The figure shows three views and two pictorial views of one solid part (mm, origin at its lowest corner). Answer the questions. A direction names the side the tool comes from. Coordinates: 2 decimals unless noted, no trailing zeros. Loops run counter-clockwise (first coordinate to the right, second up) from the corner with the lowest first, then second, coordinate; pieces in that order, holes last.
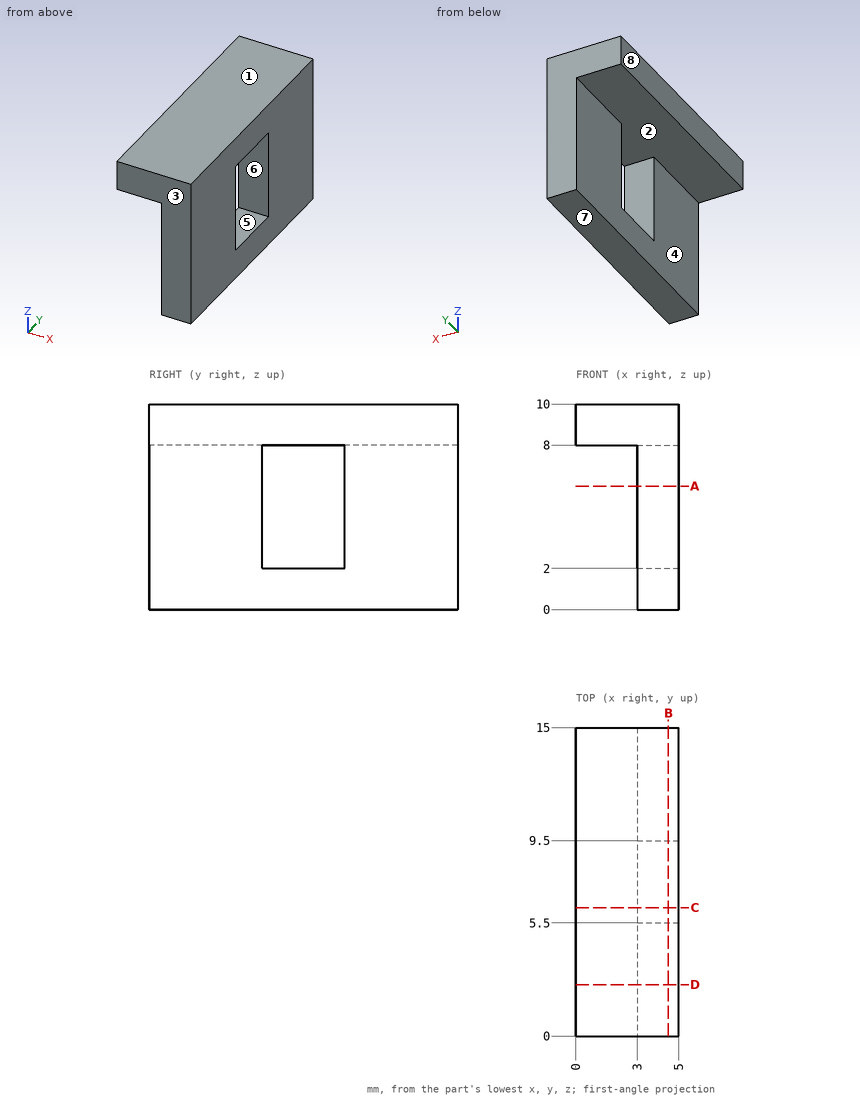
Q1. A cutting plane is placed at A-A (z = 6). Give the vertices of the cut face in (x, y).
Findings below:
outline: (3, 0) - (5, 0) - (5, 5.5) - (3, 5.5) - close; (3, 9.5) - (5, 9.5) - (5, 15) - (3, 15) - close
Q2. A cutting plane is placed at D-D (y = 2.5). Give the vertices of the cut face in (x, z), then the cut area to 3 significant figures.
Findings below:
outline: (0, 8) - (3, 8) - (3, 0) - (5, 0) - (5, 10) - (0, 10) - close
area: 26.0 mm2
Q3. Straight lines are drawn through the part: probe 1 along Y at (x, z) = (3.2, 4.5); probe 2 along X at (y, z) = (1.25, 4.5); probe 3 along Z at (x, y) = (2.95, 7.5). For each, find the intervals that lie inside material, in ascending order.
Findings below:
probe 1: y = 0 to 5.5, 9.5 to 15
probe 2: x = 3 to 5
probe 3: z = 8 to 10
Q4. Which of the six approach directions +Z, -Z, +X, -X, +Y, -Y give full straight-line access (tool end or side, diameter ignored) to the marked faces 1, 2, 3, 4 and 5?
Findings below:
face 1: +Z, +X, -X, +Y, -Y
face 2: -X
face 3: +Z, -Z, +X, -X, -Y
face 4: -Z, -X, +Y, -Y
face 5: +X, -X
Q5. A cutting plane is placed at B-B (x = 4.5). Give the vertices of the cut face in (y, z).
Findings below:
outline: (0, 0) - (15, 0) - (15, 10) - (0, 10) - close; hole (5.5, 2) - (9.5, 2) - (9.5, 8) - (5.5, 8) - close
Q6. Determine the mould class of the marked faces 6, 7 and 8 for opening direction Z: +Z half, -Z half, draft (parallel to the pull), parting line (faces both ways), or undercut.
Findings below:
face 6: undercut
face 7: -Z half
face 8: draft
Q7. Flat-ended cylindrical pins translate along their axes: pin 1 Ø1.5 at (x, y) = (0.5, 8.5) entering from -Z; pin 2 Ø2 at (y, z) = (7.5, 4.5) entering from -X; pin 3 Ø2.5 at (y, z) = (8.5, 6) entering from -X. Find the tip coordinate at first contact, or state that the pin passes through.
Findings below:
pin 1: stops at z = 8
pin 2: passes through
pin 3: stops at x = 3
Q8. A cutting plane is placed at C-C (y = 6.25). Give the vertices of the cut face in (x, z), then the cut area to 3 significant figures.
Findings below:
outline: (0, 8) - (5, 8) - (5, 10) - (0, 10) - close; (3, 0) - (5, 0) - (5, 2) - (3, 2) - close
area: 14.0 mm2
